Verification items for the finished model (mm, model axes). Face numbers are marked on the shaded views. A direction names the side the tool comes from. Round coordinates to 2 decimals unless told otherwise and drop trailing zeros. Loops run counter-clockwise (first coordinate to the right, second up) from the corner with the lowest first, then second, coordinate; pieces in that order, holes last. Notation, with made-up numbers: (40, -6.5) - (51, -6.5) arc R30 ccw to (51, 15.5) - close; hole circle Ø7 at (20, 31). An arc over 180 degrees is marked (long way). Use CSV: the item, a comma, the result in double quotes.
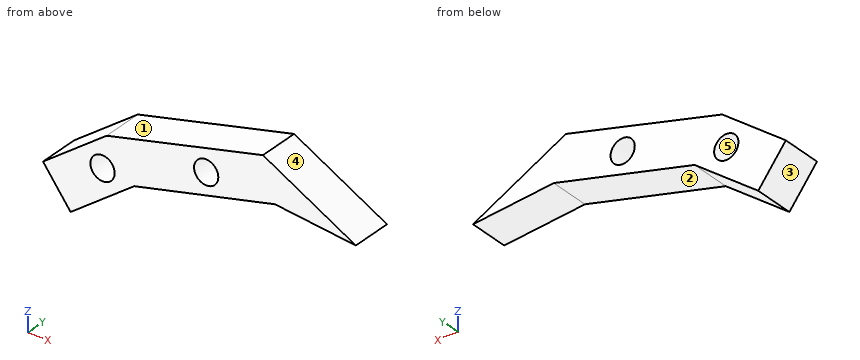
```python
from build123d import *

# Parameters (mm, degrees)
SKETCH_1_R      = 1.5
EXTRUDE_1_DEPTH = 5


with BuildPart() as part:
    # 草图1 → 凸台-拉伸1 (new body)
    with BuildSketch(Plane(origin=(0, 0, 0), x_dir=(1, 0, 0), z_dir=(0, 1, 0))):
        Polygon((-34.456184954, -3.49420181), (-26.584074683, -9.438943538), (-7.236140092, -14.504259625), (4.261211757, -8.437060891), (-5.738788243, -9.408767904), (-23.169375756, -4.917151386), (-31.041486027, 1.027590342), align=None)
        with Locations(Location((-27.087553114, -5.504570551, 0), (0, 0, 270))):
            Circle(SKETCH_1_R, mode=Mode.SUBTRACT)
        with Locations(Location((-14.25994565, -9.87219173, 0), (0, 0, 270))):
            Circle(SKETCH_1_R, mode=Mode.SUBTRACT)
    extrude(amount=EXTRUDE_1_DEPTH)


solid = part.part
```
1) Thickness scan on probe 1 along Z at (x, y) = (-26, 3.8); probe 2 along Z at (x, y) = (-28, 0.85); probe 3 along X at (y, z) = (4.4, 1.5). Record the ranges inside material, lowest first. Write a range as [from, to].
Returned:
probe 1,"z = [2.78, 4.47], [6.54, 9.59]"
probe 2,"z = [1.27, 4.31], [6.7, 8.37]"
probe 3,"x = [-32.95, -27.69]"
2) Cross-section at A-A, the plane z = 10. Record the cut outline in (x, y).
Returned:
outline,"(-24.44, 0) - (-15.75, 0) - (-15.75, 5) - (-24.44, 5) - close; (-12.77, 0) - (1.3, 0) - (1.3, 5) - (-12.77, 5) - close"
3) Cross-section at B-B, the plane x = -28. Record the cut outline in (y, z), then the cut area to 3 significant figures.
Returned:
outline,"(0, 1.27) - (5, 1.27) - (5, 4.31) - (0, 4.31) - close; (0, 6.7) - (5, 6.7) - (5, 8.37) - (0, 8.37) - close"
area,"23.6 mm²"
4) Access from +Z, -Z, +X, -X, +Y, -Y to the whole of each face (thin tool, end or side, straight path). Record for the marked faces 1 and 2.
Returned:
face 1,"+Z, -X, +Y, -Y"
face 2,"-Z, +Y, -Y"
5) Cross-section at D-D, the plane z = 2. Record the cut outline in (x, y).
Returned:
outline,"(-33.33, 0) - (-27.03, 0) - (-27.03, 5) - (-33.33, 5) - close"
6) Cross-section at C-C, the plane y = 2.95. Record the cut outline in (x, z).
Returned:
outline,"(-34.46, 3.49) - (-31.04, -1.03) - (-23.17, 4.92) - (-5.74, 9.41) - (4.26, 8.44) - (-7.24, 14.5) - (-26.58, 9.44) - close; hole circle Ø3 at (-27.09, 5.5); hole circle Ø3 at (-14.26, 9.87)"
7) Mould release check, pull along Z, two halves, no side actions. Record for the marked faces 3, 4 and 5: +Z half, -Z half, draft (parallel to the pull), parting line (faces both ways), or undercut.
Returned:
face 3,"-Z half"
face 4,"+Z half"
face 5,"undercut"
8) Gauge pin test, flat ends, axial feed: pin 1 Ø1.5 at (y, z) = (0.5, 1.5) entering from -X; pin 2 Ø1.8 at (x, z) = (-14.26, 9.87) entering from +Y; pin 3 Ø1.5 at (x, y) = (-11.5, 3.5) entering from +Z; pin 4 Ø3 at (x, y) = (-15.5, 2) entering from -Z. Record the tip position at first contact, or that the pin passes through.
Returned:
pin 1,"stops at x = -33.52"
pin 2,"passes through"
pin 3,"stops at z = 13.58"
pin 4,"stops at z = 6.51"
